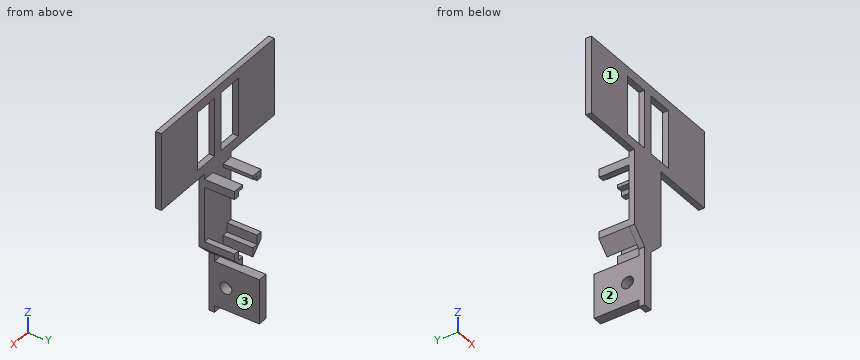
from build123d import *

# Parameters (mm, degrees)
SKETCH1_W           = 16.51
SKETCH1_H           = 39.37
BOSS_EXTRUDE1_DEPTH = 3.81
SKETCH2_W           = 6.281845558
SKETCH2_H           = 29.999999944
BOSS_EXTRUDE2_DEPTH = 30
CUT_EXTRUDE1_REACH  = 59.2
SKETCH3_R           = 4
BOSS_EXTRUDE3_DEPTH = 20


with BuildPart() as part:
    # Sketch1 → Boss-Extrude1 (new body)
    with BuildSketch(Plane(origin=(0, 0, 0), x_dir=(1, 0, 0), z_dir=(0, 1, 0))):
        Polygon((-53.975, 20.680273282), (-53.975, -31.389726718), (53.975, -31.389726718), (53.975, 20.680273282), (12.7, 20.680273282), (12.7, 71.480273282), (3.225157137, 80.955116145), (3.225157137, 120.325116145), (-3.056688421, 120.325116145), (-3.056688421, 81.123584861), (-12.7, 71.480273282), (-12.7, 20.680273282), align=None)
        with Locations((-11.43, -5.354726718)):
            Rectangle(SKETCH1_W, SKETCH1_H, mode=Mode.SUBTRACT)
        with Locations((11.43, -5.354726718)):
            Rectangle(SKETCH1_W, SKETCH1_H, mode=Mode.SUBTRACT)
    extrude(amount=BOSS_EXTRUDE1_DEPTH)

    # Sketch2 → Boss-Extrude2 (add)
    with BuildSketch(Plane(origin=(0, 3.81, 0), x_dir=(1, 0, 0), z_dir=(0, 1, 0))):
        with Locations((0.084234358, 100.640116145)):
            Rectangle(SKETCH2_W, SKETCH2_H)
    extrude(amount=BOSS_EXTRUDE2_DEPTH)

    # Sketch3 → Cut-Extrude1 (cut, up to next)
    with BuildSketch(Plane(origin=(3.225157137, 0, 0), x_dir=(0, 0, -1), z_dir=(1, 0, 0)), mode=Mode.PRIVATE) as cut_extrude1_sk1:
        with Locations((100.640116145, 11.43)):
            Circle(SKETCH3_R)
    cut_extrude1_tool1 = extrude(cut_extrude1_sk1.sketch, amount=-CUT_EXTRUDE1_REACH, mode=Mode.PRIVATE) & part.part
    add(cut_extrude1_tool1.solids().sort_by_distance((3.225157, 11.43, -100.640116))[0], mode=Mode.SUBTRACT)

    # Sketch6 → Boss-Extrude3 (add)
    with BuildSketch(Plane(origin=(0, 3.81, 0), x_dir=(1, 0, 0), z_dir=(0, 1, 0))):
        Polygon((-8.128, 24.319391954), (-4.952973996, 24.319391954), (-4.952973996, 26.561602149), (-8.829142948, 26.561602149), (-8.829142948, 29.779456866), (-12.7, 29.779456866), (-12.7, 24.319391954), align=None)
        Polygon((12.7, 24.319391954), (8.128, 24.319391954), (4.952973996, 24.319391954), (4.952973996, 26.561602149), (8.829142948, 26.561602149), (8.829142948, 29.779456866), (12.7, 29.779456866), align=None)
        Polygon((-4.952973996, 79.227299287), (-12.7, 71.480273282), (-12.7, 66.743012955), (-8.829142948, 66.743012955), (-8.829142948, 72.988681503), (-4.952973996, 72.988681503), align=None)
        Polygon((4.952973996, 72.988681503), (4.952973996, 79.227299287), (12.7, 71.480273282), (12.7, 66.743012955), (8.829142948, 66.743012955), (8.829142948, 72.988681503), align=None)
    extrude(amount=BOSS_EXTRUDE3_DEPTH)


solid = part.part
Build history of the part. All positions in model axes, mm. Face numbers are marked on the shaded views. A direction names the side the tool comes from. Give positions to 0.01 mm unless a question says otherwise; leave off trailing zeros. Write each loop counter-clockwise with the first axis right and the second up, starting at its lowest first coordinate (ties: lowest second). Pieces come first, ordered by that corner, then holes. Notation, with made-up numbers: (30, -17.5) - (37, -17.5) arc R22 cw to (37, -7.5) - close; hole circle Ø4 at (72.25, -3.5). An arc over 180 degrees is marked (long way). Use one line per item in the form item = value. Start each with the question number.
1. Band-saw the part on B-B on x = 18. Write the cut outline in (y, z), plus the area to 3 significant figures.
2. Drop flat-ended pins along their axis: pin 1 Ø1.6 at (x, z) = (-10, -27.5) entering from +Y; pin 2 Ø6 at (y, z) = (14.5, -79) entering from +X; pin 3 Ø17 at (y, z) = (20.5, -91) entering from -X. Give the stop position or say it passes through.
3. Band-saw the part on C-C on z = 6. Write the cut outline in (x, y) (3 decimals).
4. Band-saw the part on D-D on x = 0.5. Write the cut outline in (y, z), plus the area to 3 significant figures.
5. Probe line 1 (X direction, y = 8, z = -68.5); line 2 (Z direction, x = 0, y = 11); line 3 (X direction, y = 27, z = -93.5). List the from-to ranges inside material, lowest first. Write a range as [from, to].
6. 3-axis set-ups, long thin cutter, end or side, ignore diameter. For the marked faces 1, 2 and 3: which of +Z, -Z, +X, -X, +Y, -Y reach the whole face in a straight line?
7. Band-saw the part on A-A on y = 18. Write the cut outline in (x, z).
Conclusion:
q1.outline = (0, -20.68) - (3.81, -20.68) - (3.81, -14.33) - (0, -14.33) - close; (0, 25.04) - (3.81, 25.04) - (3.81, 31.39) - (0, 31.39) - close
q1.area = 48.4 mm²
q2.pin_1 = 23.81
q2.pin_2 = 8.18
q2.pin_3 = -3.06
q3.outline = (-53.975, 0) - (-19.685, 0) - (-19.685, 3.81) - (-53.975, 3.81) - close; (-3.175, 0) - (3.175, 0) - (3.175, 3.81) - (-3.175, 3.81) - close; (19.685, 0) - (53.975, 0) - (53.975, 3.81) - (19.685, 3.81) - close
q4.outline = (0, -120.33) - (3.81, -120.33) - (3.81, -115.64) - (33.81, -115.64) - (33.81, -85.64) - (3.81, -85.64) - (3.81, 31.39) - (0, 31.39) - close; hole circle Ø8 at (11.43, -100.64)
q4.area = 1,430 mm²
q5.line_1 = [-12.7, -8.83], [8.83, 12.7]
q5.line_2 = [-115.64, -104.62], [-96.66, -85.64]
q5.line_3 = [-3.06, 3.23]
q6.face_1 = +Z, -Z, +X, -X, -Y
q6.face_2 = -Z, -X, +Y, -Y
q6.face_3 = -Z, +X, +Y, -Y
q7.outline = (-12.7, -71.48) - (-4.95, -79.23) - (-4.95, -72.99) - (-8.83, -72.99) - (-8.83, -66.74) - (-12.7, -66.74) - close; (-12.7, -29.78) - (-8.83, -29.78) - (-8.83, -26.56) - (-4.95, -26.56) - (-4.95, -24.32) - (-12.7, -24.32) - close; (-3.06, -115.64) - (3.23, -115.64) - (3.23, -85.64) - (-3.06, -85.64) - close; (4.95, -79.23) - (12.7, -71.48) - (12.7, -66.74) - (8.83, -66.74) - (8.83, -72.99) - (4.95, -72.99) - close; (4.95, -26.56) - (8.83, -26.56) - (8.83, -29.78) - (12.7, -29.78) - (12.7, -24.32) - (4.95, -24.32) - close
